The model under review builds one solid part; all positions refer to its coordinate system, in mm. A direction names the side the tool comes from. Coordinates: 2 decimals unless noted, no trailing zeros. Write each loop counter-clockwise with the first axis right and the second up, starting at its lowest first coordinate (ties: lowest second). Pieces come first, ordered by that corner, then holes. Notation, with made-up numbers: M 14.25,24 L 30.25,24 A31 cw 30.25,56 Z; hole C 39,-1.75 d3. An arc over 180 degrees is marked long. Answer as a JSON object with one key per item and string values.
```python
from build123d import *

# Parameters (mm, degrees)
SKETCH1_W               = 34.925
SKETCH1_H               = 25.4
BOSS_EXTRUDE1_DEPTH     = 2.54
CUT_EXTRUDE3_DEPTH      = 44.259302179
CUT_EXTRUDE3_DEPTH_BACK = 44.259302179
SKETCH2_R               = 1.74625
SKETCH5_R               = 1.1303
CUT_EXTRUDE4_DEPTH      = 44.259302179
SKETCH6_W               = 10.16
SKETCH6_H               = 21.59
BOSS_EXTRUDE2_DEPTH     = 2.54
FILLET1_R               = 2.54
FILLET2_R               = 1.5875
FILLET3_R               = 2.54
SKETCH8_W               = 6.597299276
SKETCH8_H               = 1.6002
CUT_EXTRUDE6_DEPTH      = 2.54


with BuildPart() as part:
    # Sketch1 → Boss-Extrude1 (new body)
    with BuildSketch(Plane(origin=(0, 0, 0), x_dir=(1, 0, 0), z_dir=(0, 1, 0))):
        with Locations((17.4625, 12.7)):
            Rectangle(SKETCH1_W, SKETCH1_H)
    extrude(amount=BOSS_EXTRUDE1_DEPTH)

    # Sketch2 → Cut-Extrude3 (cut, two sides: drawn at the far end of the back side and taken through both)
    with BuildSketch(Plane(origin=(0, 2.54, 0), x_dir=(1, 0, 0), z_dir=(0, 1, 0)).offset(-CUT_EXTRUDE3_DEPTH_BACK)):
        with Locations(Location((3.81, 18.415, 0), (0, 0, 90))):
            Circle(SKETCH2_R)
        with Locations(Location((3.81, 6.985, 0), (0, 0, 90))):
            Circle(SKETCH2_R)
    extrude(amount=CUT_EXTRUDE3_DEPTH + CUT_EXTRUDE3_DEPTH_BACK, mode=Mode.SUBTRACT)

    # Sketch5 → Cut-Extrude4 (cut, through all)
    with BuildSketch(Plane(origin=(0, 2.54, 0), x_dir=(1, 0, 0), z_dir=(0, 1, 0))):
        with Locations(Location((31.75, 20.32, 0), (0, 0, 270))):
            Circle(SKETCH5_R)
        with Locations(Location((31.75, 5.08, 0), (0, 0, 90))):
            Circle(SKETCH5_R)
    extrude(amount=-CUT_EXTRUDE4_DEPTH, mode=Mode.SUBTRACT)

    # Sketch6 → Boss-Extrude2 (add)
    with BuildSketch(Plane(origin=(0, 2.54, 0), x_dir=(1, 0, 0), z_dir=(0, 1, 0))):
        with Locations((31.75, 36.195)):
            Rectangle(SKETCH6_W, SKETCH6_H)
    extrude(amount=-BOSS_EXTRUDE2_DEPTH)

    # Fillet1
    # the kernel refuses this fillet: 2.54 mm, written as the material it adds along each edge
    with BuildSketch(Plane(origin=(26.67, 2.54, -25.4), x_dir=(-1, 0, 0), z_dir=(0, -1, 0))) as fillet1_piece_1:
        with BuildLine():
            CenterArc((FILLET1_R, FILLET1_R), FILLET1_R, 180, 90)
            Line((0, FILLET1_R), (-FILLET1_R * 0.02, FILLET1_R))
            Line((-FILLET1_R * 0.02, FILLET1_R), (-FILLET1_R * 0.02, -FILLET1_R * 0.02))
            Line((-FILLET1_R * 0.02, -FILLET1_R * 0.02), (FILLET1_R, -FILLET1_R * 0.02))
            Line((FILLET1_R, -FILLET1_R * 0.02), (FILLET1_R, 0))
        make_face()
    extrude(amount=2.54)
    with BuildSketch(Plane(origin=(34.925, 0, -25.4), x_dir=(0, 0, 1), z_dir=(0, 1, 0))) as fillet1_piece_2:
        with BuildLine():
            CenterArc((2.459344425, 2.54), FILLET1_R, 194.477512186, 75.522487814)
            Line((0, 1.905), (-0.049186888, 1.8923))
            ThreePointArc((-0.049186888, 1.8923), (-0.0508, 0.9525), (-0.0508, 0))
            Line((-0.0508, 0), (0, -0.0508))
            Line((0, -0.0508), (2.459344425, -0.0508))
            Line((2.459344425, -0.0508), (2.459344425, 0))
        make_face()
    extrude(amount=2.54)

    # Fillet2
    fillet2_edges = [part.edges().sort_by_distance(p)[0] for p in [
        (26.67, 1.27, -46.99),
        (36.83, 1.27, -46.99),
        (36.83, 1.27, -25.4),
    ]]
    fillet(fillet2_edges, radius=FILLET2_R)

    # Fillet3
    fillet3_edges = [part.edges().sort_by_distance(p)[0] for p in [
        (0, 1.27, -25.4),
        (34.925, 1.27, 0),
        (0, 1.27, 0),
    ]]
    fillet(fillet3_edges, radius=FILLET3_R)

    # Sketch8 → Cut-Extrude6 (cut)
    with BuildSketch(Plane(origin=(0, 2.54, 0), x_dir=(1, 0, 0), z_dir=(0, 1, 0))):
        with Locations((31.75, 44.45)):
            Rectangle(SKETCH8_W, SKETCH8_H)
    extrude(amount=-CUT_EXTRUDE6_DEPTH, mode=Mode.SUBTRACT)


solid = part.part
```
(1) For faces 5 (the face through (26.67, 1, -37)), 6 (the face through (35.049, 1, -44)), 7 (the face through (36.83, 1, -36)), list the 3-axis set-ups (+Z, -Z, +X, -X, +Y, -Y) from which the entire face can be reached by the end or side of a thin tool; tool diameter is ignored.
Results list:
{"face 5": "-Z, -X, +Y, -Y", "face 6": "+Y, -Y", "face 7": "+Z, -Z, +X, +Y, -Y"}
(2) Draft analysis for pull direction Z (two halves, no side actions). For faces 1 (the face through (19, 2.54, -18)), 2 (the face through (3.73, 1.25, -16.67)), 3 (the face through (0.724, 1.288, -24.636)), 4 (the face through (28.451, 1, -44)), state which applies: released by +Z, released by -Z, zero draft, split by the parting line, or undercut.
Results list:
{"face 1": "zero draft", "face 2": "undercut", "face 3": "released by -Z", "face 4": "undercut"}
(3) Add section B-B on y = 0.9. Count the separate pieces of the cut face and the enclosed holes in it, and give its area (3 significant figures).
Results list:
{"separate pieces": "1", "enclosed holes": "5", "area": "1,070 mm²"}
(4) Add section C-C on x = 3.81. Give the boundary of the cut face in (y, z).
Results list:
{"outline": "M 0,-25.4 L 2.54,-25.4 L 2.54,-20.16 L 0,-20.16 Z; M 0,-16.67 L 2.54,-16.67 L 2.54,-8.73 L 0,-8.73 Z; M 0,-5.24 L 2.54,-5.24 L 2.54,0 L 0,0 Z"}
(5) Wall thickness on line 1 along X through (y, z) = (2.05, -20.32) (3 decimals); line 2 along X through (y, z) = (0.45, -30); line 3 along Z through (x, y) = (32.5, 1.5): over which ranges is each line inside the solid? List them lowest first. Write a range as from..to.
Results list:
{"line 1": "0..30.62, 32.88..34.925", "line 2": "26.67..36.83", "line 3": "-46.99..-45.25, -43.65..-21.17, -19.47..-5.93, -4.23..0"}
(6) Add section D-D on z = -40.5. Give the boundary of the cut face in (x, y).
Results list:
{"outline": "M 26.67,0 L 36.83,0 L 36.83,2.54 L 26.67,2.54 Z"}
(7) Add section A-A on x = 31.75. Give the boundary of the cut face in (y, z), and give its area (3 significant figures).
Results list:
{"outline": "M 0,-46.99 L 2.54,-46.99 L 2.54,-45.25 L 0,-45.25 Z; M 0,-43.65 L 2.54,-43.65 L 2.54,-21.45 L 0,-21.45 Z; M 0,-19.19 L 2.54,-19.19 L 2.54,-6.21 L 0,-6.21 Z; M 0,-3.95 L 2.54,-3.95 L 2.54,0 L 0,0 Z", "area": "104 mm²"}
(8) For pin 1 Ø3 at (x, z) = (3.81, -18.415) entering from +Y; pin 2 Ø0.8 at (y, z) = (1, -33) entering from -X; pin 3 Ø1.3 at (x, y) = (12.5, 2) entering from -Z, all flat-tipped, find the tip position at first contact; note any pin that passes through.
Results list:
{"pin 1": "through", "pin 2": "x = 26.67", "pin 3": "z = -25.4"}
